Build history of the part. All positions in model axes, mm. A direction names the side the tool comes from. Round coordinates to 2 decimals unless told otherwise and drop trailing zeros. Write each loop counter-clockwise with the first axis right and the second up, starting at its lowest first coordinate (ties: lowest second). Pieces come first, ordered by that corner, then holes.
1) Saw through at D-D (z = 56.5). State how many separate pieces and enclosed holes the cut face has, plus the area to 3 significant figures.
2) Saw through at A-A (x = 0). Write the cut outline in (y, z) (3 decimals).
3) Saw through at C-C (x = -14). Write the cut outline in (y, z) (3 decimals), plus the area to 3 significant figures.
4) Pull direction X, two halves, no side cores. Call faces 1 (the cylindrical face through (-4.918, 13.341, 32.045)), 2 (the flat face through (0, -13.575, 32)), 3 (the flat face through (-11.604, 7.052, 32.045)): +X half, -X half, draft (parallel to the pull), parting line (faces both ways), or undercut.
5) Flat gauge pins, fed straight in: pin 1 (2 mm diameter, centred on x = -16, z = 19, fed in from +Y); pin 2 (3 mm diameter, centred on x = 11.5, z = 36, fed in from +Y); pin 3 (3 mm diameter, centred on y = 16.5, z = 14.5, fed in from +X); pin 4 (18.5 mm diameter, centred on x = 0, y = 0, fed in from +Z). Where does each tip first touch, or does it go through?
6) Which spindle directions (+Z, -Z, +X, -X, +Y, -Y) get a long thin tool onto all of the face, cutting with end or side? Do faces 4 (the cylindrical face through (11.73, -6.83, 32.04)), 5 (the flat face through (-9, 8, 0)). Say none if no direction does.
7) Wall check: probe 1 along X at (y, z) = (20.5, 57); probe 2 along Y at (x, z) = (-16, 35) (3 decimals); probe 3 along X at (y, z) = (18.5, 61.5). Give the ranges that are in metal, low to high.
8) Saw through at B-B (y = 20). Write the cut outline in (x, z).
from build123d import *

# Parameters (mm, degrees)
F0_R     = 11.575
F1_DEPTH = 65


with BuildPart() as f1:
    # F0 (on Top) → F1 (new body)
    with BuildSketch(Plane.XY):
        with BuildLine():
            Line((11.756295, 6.7875), (0.866025, 25.65))
            ThreePointArc((0.866025, 25.65), (0, 26.15), (-0.866025, 25.65))
            Line((-0.866025, 25.65), (-22.646564, -12.075))
            ThreePointArc((-22.646564, -12.075), (-22.646564, -13.075), (-21.780539, -13.575))
            Line((-21.780539, -13.575), (21.780539, -13.575))
            ThreePointArc((21.780539, -13.575), (22.646564, -13.075), (22.646564, -12.075))
            Line((22.646564, -12.075), (11.756295, 6.7875))
        make_face()
        with BuildLine():
            ThreePointArc((-18.316437, -11.575), (-19.182463, -11.075), (-19.182463, -10.075))
            Line((-19.182463, -10.075), (-15.039222, -2.898696))
            ThreePointArc((-15.039222, -2.898696), (-14.029572, -2.409064), (-13.200764, -3.165509))
            ThreePointArc((-13.200764, -3.165509), (-11.756295, -6.7875), (-9.341794, -9.849443))
            ThreePointArc((-9.341794, -9.849443), (-9.101096, -10.945434), (-10.029955, -11.575))
            Line((-10.029955, -11.575), (-18.316437, -11.575))
        make_face(mode=Mode.SUBTRACT)
        Circle(F0_R, mode=Mode.SUBTRACT)
        with BuildLine():
            ThreePointArc((19.182463, -10.075), (19.182463, -11.075), (18.316437, -11.575))
            Line((18.316437, -11.575), (10.029955, -11.575))
            ThreePointArc((10.029955, -11.575), (9.101096, -10.945434), (9.341794, -9.849443))
            ThreePointArc((9.341794, -9.849443), (11.756295, -6.7875), (13.200764, -3.165509))
            ThreePointArc((13.200764, -3.165509), (14.029572, -2.409064), (15.039222, -2.898696))
            Line((15.039222, -2.898696), (19.182463, -10.075))
        make_face(mode=Mode.SUBTRACT)
        with BuildLine():
            ThreePointArc((-0.866025, 21.65), (0, 22.15), (0.866025, 21.65))
            Line((0.866025, 21.65), (5.009266, 14.473696))
            ThreePointArc((5.009266, 14.473696), (4.928476, 13.354498), (3.858971, 13.014952))
            ThreePointArc((3.858971, 13.014952), (0, 13.575), (-3.858971, 13.014952))
            ThreePointArc((-3.858971, 13.014952), (-4.928476, 13.354498), (-5.009266, 14.473696))
            Line((-5.009266, 14.473696), (-0.866025, 21.65))
        make_face(mode=Mode.SUBTRACT)
    extrude(amount=F1_DEPTH)


solid = f1.part
Evaluation:
1. separate pieces: 1
1. enclosed holes: 4
1. area: 371 mm2
2. outline: (-13.575, 0) - (-11.575, 0) - (-11.575, 65) - (-13.575, 65) - close; (11.575, 0) - (13.575, 0) - (13.575, 65) - (11.575, 65) - close; (22.15, 0) - (26.15, 0) - (26.15, 65) - (22.15, 65) - close
3. outline: (-13.575, 0) - (-11.575, 0) - (-11.575, 65) - (-13.575, 65) - close; (-2.414, 0) - (2.901, 0) - (2.901, 65) - (-2.414, 65) - close
3. area: 475 mm2
4. face 1: undercut
4. face 2: draft
4. face 3: -X half
5. pin 1: stops at y = 1.17
5. pin 2: stops at y = 9.83
5. pin 3: stops at x = 7.01
5. pin 4: passes through
6. face 4: +Z, -Z
6. face 5: -Z, +X, -X, +Y, -Y
7. probe 1: x = -3.84 to -1.53, 1.53 to 3.84
7. probe 2: y = -13.575 to -11.575, -4.563 to -0.563
7. probe 3: x = -4.99 to -2.68, 2.68 to 4.99
8. outline: (-4.13, 0) - (-1.82, 0) - (-1.82, 65) - (-4.13, 65) - close; (1.82, 0) - (4.13, 0) - (4.13, 65) - (1.82, 65) - close
